```python
from build123d import *

# Parameters (mm, degrees)
ZAOBLIT1_R = 1


with BuildPart() as part:
    # Skica1 → Rotovat1 (revolve)
    with BuildSketch(Plane.XY, mode=Mode.PRIVATE) as rotovat1_sk:
        Polygon((-1.5, 0), (-8, 0), (-6.5, 7.8), (-3, 7.8), (-3, 4), (-1.5, 4), align=None)
    revolve(rotovat1_sk.sketch.rotate(Axis((0, 16.170731707, 0), (0, -1, 0)), 270), axis=Axis((0, 16.170731707, 0), (0, -1, 0)))

    # Zaoblit1
    zaoblit1_edges = [part.edges().sort_by_distance(p)[0] for p in [
        (0, 7.8, -6.5),
    ]]
    fillet(zaoblit1_edges, radius=ZAOBLIT1_R)


solid = part.part
```
Geometry: final body of the model. Coordinates: model frame, mm. A direction names the side the tool comes from. Give positions to 0.01 mm unless a question says otherwise; leave off trailing zeros. Loops run counter-clockwise (first coordinate to the right, second up) from the corner with the lowest first, then second, coordinate; pieces in that order, holes last. Notation, with made-up numbers: (11, -7.75) -> (46, -7.75) arc R11 ccw to (46, 10.25) -> close; hole circle Ø11 at (73.25, 32.5). An arc over 180 degrees is marked (long way). Use one line per item in the form item = value.
Item 1: Section query A-A on z = 0. Output: boundary loops of the cut face in (x, y), and give its area (3 significant figures).
A:
outline = (-8, 0) -> (-1.5, 0) -> (-1.5, 4) -> (-3, 4) -> (-3, 7.8) -> (-5.67, 7.8) arc R1 ccw to (-6.66, 6.99) -> close; (1.5, 0) -> (8, 0) -> (6.66, 6.99) arc R1 ccw to (5.67, 7.8) -> (3, 7.8) -> (3, 4) -> (1.5, 4) -> close
area = 78.0 mm^2
Item 2: Line query: probe 1 along X at (y, z) = (5.7, 0); probe 2 along X at (y, z) = (6, -2.75); probe 3 along Z at (x, y) = (0.5, 1.5). Output: solid intervals per line, ascending.
A:
probe_1 = -6.9 to -3, 3 to 6.9
probe_2 = -6.27 to -1.2, 1.2 to 6.27
probe_3 = -7.7 to -1.41, 1.41 to 7.7
Item 3: Section query B-B on x = 0. Output: boundary loops of the cut face in (y, z), and give its area (3 significant figures).
A:
outline = (0, -8) -> (6.99, -6.66) arc R1 ccw to (7.8, -5.67) -> (7.8, -3) -> (4, -3) -> (4, -1.5) -> (0, -1.5) -> close; (0, 1.5) -> (4, 1.5) -> (4, 3) -> (7.8, 3) -> (7.8, 5.67) arc R1 ccw to (6.99, 6.66) -> (0, 8) -> close
area = 78.0 mm^2
Item 4: Section query D-D on y = 3.5. Output: boundary loops of the cut face in (x, z), and give its area (3 significant figures).
A:
outline = circle Ø14.65 at (0, 0); hole circle Ø3 at (0, 0)
area = 162 mm^2
Item 5: Access query for faces 4 (the face through (0, 0, -2)), 5 (the face through (-0.9, 5.87, 2.86)). Directions: +Z, -Z, +X, -X, +Y, -Y. A direction counts if a zero-diameter tool reaches every point of the face in a straight line with its end or side. Return the directions, or none.
A:
face_4 = +Z, -Z, +X, -X, -Y
face_5 = +Y
Item 6: Section query C-C on y = 1. Output: boundary loops of the cut face in (x, z), and give its area (3 significant figures).
A:
outline = circle Ø15.62 at (0, 0); hole circle Ø3 at (0, 0)
area = 184 mm^2
Item 7: Pin query (flat end, axial travel): P1, Ø3, axis at x = -0.5, z = 1.5, coming from the +Y side; P2, Ø2.5, axis at x = 0, z = 0, coming from the +Y side. Return the tip coordinate at first contact, or that it passes through.
A:
P1 = 7.8
P2 = through
Item 8: Draft query along Z for faces 1 (the face through (2.4, 7.8, 2.4)), 2 (the face through (-2.109, 5.096, 6.696)), 3 (the face through (1.3, 4, 1.3)). Return one class per face: pulls with the +Z half, pulls with the -Z half, needs draft (parallel to the pull), parting line crosses it, or undercut.
A:
face_1 = needs draft
face_2 = parting line crosses it
face_3 = undercut
